Source: CAD feature listing. Evaluate the final solid. Frame: model axes, mm. A direction names the side the tool comes from. Give positions to 0.01 mm unless a question says otherwise; leave off trailing zeros. Order: outer loops, then holes, each group sorted by start corner. A loop starts at its lowest first (then second) coordinate and runs counter-clockwise, first axis right, second up. Notation, with made-up numbers: (78, -6) - (113, -6) arc R12 cw to (113, 2) - close; hole circle Ø9 at (16, 79.5). An arc over 180 degrees is marked (long way). Use CSV: the item, a comma, the result in double quotes.
Autodesk Inventor part; units mm, degrees
ref_plane "PoleBase Plane" through (57.325, 9.4828, 4.9562) normal (0, 0.9996, -0.03) x (-1, 0, 0)
ref_plane "YZ Plane" through (0, 0, 0) normal (1, 0, 0) x (0, 1, 0)
ref_plane "XZ Plane" through (0, 0, 0) normal (0, 1, 0) x (-1, 0, 0)
sketch "Spacebar base" plane through (0, 0, 0) normal (0, 1, 0) x (-1, 0, 0)
  line L0 (58.825, 9.05) -> (-58.825, 9.05)
  line L1 (-58.825, 9.05) -> (-58.825, -9.05)
  line L2 (-58.825, -9.05) -> (58.825, -9.05)
  line L3 (58.825, -9.05) -> (58.825, 9.05)
  line L4 (58.825, 9.05) -> (-58.825, -9.05) construction
  line L5 (-58.825, 9.05) -> (58.825, -9.05) construction
  point P0 (0, 0)
  dimension "d0" = 117.65
  dimension "d1" = 18.1
extrude "Spacebar Bulk" add sketch "Spacebar base" along normal blind 11
sketch "Curve Profile" plane through (58.825, 0, 9.05) normal (1, 0, 0) x (0, 0, -1)
  line L0 (0, 0) -> (18.1, 0)
  line L1 (0, 0) -> (2.9474, 11)
  line L2 (0, 11) -> (18.1, 11)
  line L3 (18.1, 0) -> (18.1, 11)
  arc A0 (18.1, 8) -> (2.9474, 11) centre (2.9474, -28.7667) ccw
  line L4 (0, 0) -> (0, 11)
  line L5 (18.1, 8) -> (18.1, 0)
  line L6 (18.1, 0) -> (0, 0)
  point P0 (9.05, 0)
  dimension "d4" = 15
  dimension "d9" = 8
extrude "Curve Cutaway" cut sketch "Curve Profile" against normal up to surface (117.65 mm away) contours L1 A0 L3 L0 keep common part
shell "Inner Shell" thickness 1.5 removed faces 1 at (19.6083, 0, 3.0167)
ref_plane "PoleBase Plane" through (57.325, 9.4828, 4.9562) normal (0, 0.9996, -0.03) x (-1, 0, 0)
sketch "Center Circle" plane through (57.325, 9.4828, 4.9562) normal (0, 0.9996, -0.03) x (-1, 0, 0)
  circle A0 centre (57.325, -5.238) radius 2.77
  dimension "d11" = 5.54
extrude "Pole Extrusion" add sketch "Center Circle" against normal up to surface surface through (0, 0, 0) normal (0, 1, 0)
sketch "Sketch4" plane through (0, 0, 0) normal (0, -1, 0) x (1, 0, 0)
  line L0 (-2.2, 0.675) -> (2.2, 0.675)
  line L1 (2.2, 0.675) -> (2.2, -0.675)
  line L2 (2.2, -0.675) -> (-2.2, -0.675)
  line L3 (-2.2, -0.675) -> (-2.2, 0.675)
  line L4 (-2.2, 0.675) -> (2.2, -0.675) construction
  line L5 (2.2, 0.675) -> (-2.2, -0.675) construction
  line L6 (0.675, 2.2) -> (-0.675, 2.2)
  line L7 (-0.675, 2.2) -> (-0.675, -2.2)
  line L8 (-0.675, -2.2) -> (0.675, -2.2)
  line L9 (0.675, -2.2) -> (0.675, 2.2)
  line L10 (0.675, 2.2) -> (-0.675, -2.2) construction
  line L11 (-0.675, 2.2) -> (0.675, -2.2) construction
  point P0 (0, 0)
  dimension "d14" = 4.4
  dimension "d15" = 1.35
  dimension "d16" = 1.35
  dimension "d17" = 4.4
extrude "Extrusion4" cut sketch "Sketch4" against normal blind 5
equation "\"d0\" = b_space"
equation "\"d1\" = k_width"
equation "\"d10\" = k_wthick"
equation "\"d11\" = k_poledia"
equation "\"d14\" = k_cmxl"
equation "\"d15\" = k_cmxw"
equation "\"d16\" = k_cmxw"
equation "\"d17\" = k_cmxl"
equation "\"k_width\" = 18.1"
equation "\"k_height\" = 18"
equation "\"k_height_t\" = 16"
equation "\"k_taper1\" = 1.5"
equation "\"k_taper2\" = 0.5"
equation "\"k_staper\" = 1"
equation "\"k_sradius\" = 4"
equation "\"k_ltaper\" = 1.5"
equation "\"k_lradius\" = 6"
equation "\"k_radius\" = 6"
equation "\"k_wthick\" = 1.5"
equation "\"k_ribthick\" = 1.5"
equation "\"k_ribheight\" = 5"
equation "\"k_poleoff\" = 2.2625"
equation "\"k_poledia\" = 5.54"
equation "\"k_cmxw\" = 1.35"
equation "\"k_cmxl\" = 4.4"
equation "\"s_bwidth\" = 15.6"
equation "\"s_poleh\" = 3.6"
equation "\"s_polebw\" = 5.5"
equation "\"s_polebl\" = 7"
equation "\"b_pad\" = 1"
equation "\"b_tab\" = 27.15"
equation "\"b_caps\" = 31.675"
equation "\"b_lshift\" = 40.725"
equation "\"b_rshift\" = 49.775"
equation "\"b_ctrl\" = 22.625"
equation "\"b_space\" = 117.65"
equation "\"b_width\" = 286.5"
equation "\"b_height\" = 77.4"
properties part number "spacebar-keycap_mockup_cherrymx"
Item 1: Material intervals for line 1 (X direction, y = 6.5, z = -0.5) (3 decimals); line 2 (X direction, y = 1.75, z = 2.25) (3 decimals); line 3 (X direction, y = 8.5, z = 4.5) (3 decimals), sorted ascending. Write a range as from..to.
Filled in:
line 1,"x = -58.825..-57.325, -2.753..2.753, 57.325..58.825"
line 2,"x = -58.825..-57.325, -1.542..1.542, 57.325..58.825"
line 3,"x = -58.825..-57.325, 57.325..58.825"
Item 2: Section C-C on y = 2. Count the separate pieces of the cut face and the enclosed holes in it, then the cut area to 3 significant figures.
Filled in:
separate pieces,"2"
enclosed holes,"2"
area,"417 mm2"
Item 3: First-contact query: pin 1 (2 mm diameter, centred on x = 28, y = 2.5, fed in from +Z); pin 2 (6 mm diameter, centred on x = -2.5, z = 0, fed in from +Y); pin 3 (2 mm diameter, centred on x = -23.5, z = -2, fed in from +Y). Flat tips, straight axial feed; report the tip coordinate or a pass-through.
Filled in:
pin 1,"stops at z = 8.65"
pin 2,"stops at y = 10.88"
pin 3,"stops at y = 10.36"
Item 4: Section A-A on x = 16.5. Return the cut outline in (y, z), then the cut area to 3 significant figures.
Filled in:
outline,"(0, -9.05) - (8, -9.05) arc R39.77 ccw to (11, 6.1) - (0, 9.05) - (0, 7.5) - (9.48, 4.96) arc R38.27 cw to (6.98, -7.55) - (0, -7.55) - close"
area,"48.4 mm2"
Item 5: Section B-B on z = -5.5. Return the cut outline in (x, y) (3 decimals).
Filled in:
outline,"(-58.825, 0) - (-57.325, 0) - (-57.325, 7.699) - (57.325, 7.699) - (57.325, 0) - (58.825, 0) - (58.825, 9.27) - (-58.825, 9.27) - close"
Item 6: Mould query, pull axis X, two halves, no side actions, for faces 1 (the flat face through (58.825, 5, 0)), 2 (the flat face through (0, 0, 8)), 3 (the flat face through (0.803, 4.675, 6.244)). Classes: released by +X, released by -X, zero draft, split by the parting line, or undercut.
Filled in:
face 1,"released by +X"
face 2,"zero draft"
face 3,"undercut"
Item 7: Set-up query: faces 4 (the cylindrical face through (-1.489, 4.717, 2.196)), 5 (the flat face through (1, 3, -7.55)), 6 (the flat face through (-58.825, 5, 0)). Return all of +Z, -Z, +X, -X, +Y, -Y with unobstructed straight access to the full face (end or side cutting, diameter ignored); none if empty.
Filled in:
face 4,"none"
face 5,"-Y"
face 6,"+Z, -Z, -X, +Y, -Y"
